Work out the finished part from the listing and answer in its coordinate system (mm). Round coordinates to 2 decimals unless told otherwise and drop trailing zeros. Order: outer loops, then holes, each group sorted by start corner. A loop starts at its lowest first (then second) coordinate and runs counter-clockwise, first axis right, second up. Notation, with made-up numbers: M -14.75,-38 L -4.75,-38 A24 cw -4.75,-17 Z; hole C -20.75,-18.75 d9. An arc over 180 degrees is marked long. Answer as a JSON object with one key per item and string values. Group by question number.
from build123d import *

# Parameters (mm, degrees)
SKETCH1_R           = 15
SKETCH1_R_2         = 13
SKETCH1_R_3         = 11.1
BOSS_EXTRUDE1_DEPTH = 6
SKETCH1_3_R         = 15
SKETCH1_3_R_2       = 13
CUT_EXTRUDE1_DEPTH  = 3.5
CHAMFER1_SIZE       = 2


with BuildPart() as part:
    # Sketch1 → Boss-Extrude1 (new, symmetric)
    # profile 1 of 2: a face of its own
    with BuildSketch(Plane.XY):
        Circle(SKETCH1_R)
        Circle(SKETCH1_R_2, mode=Mode.SUBTRACT)
    # profile 2 of 2: a face of its own
    with BuildSketch(Plane.XY):
        Circle(SKETCH1_R_2)
        Circle(SKETCH1_R_3, mode=Mode.SUBTRACT)
    extrude(amount=BOSS_EXTRUDE1_DEPTH, both=True)

    # Sketch1<3> → Cut-Extrude1 (cut, symmetric)
    with BuildSketch(Plane.XY):
        Circle(SKETCH1_3_R)
        Circle(SKETCH1_3_R_2, mode=Mode.SUBTRACT)
    extrude(amount=CUT_EXTRUDE1_DEPTH, both=True, mode=Mode.SUBTRACT)

    # Chamfer1
    chamfer1_edges = [part.edges().sort_by_distance(p)[0] for p in [
        (-15, 0, -3.5),
        (-15, 0, 3.5),
    ]]
    chamfer(chamfer1_edges, length=CHAMFER1_SIZE - 0.0001)  # a hair under: the kernel refuses the full size


solid = part.part
Item 1: Find section C-C (z = 1). Give the vertices of the cut face in (x, y), and give its area (3 significant figures).
Item 2: The mould has two halves that part along Z. Classify faces 1 (the cylindrical face through (-10.316, -7.91, -0.049)), 2 (the flat face through (2.2, 11.2, -6)), 3 (the cylindrical face through (-14.985, 0.66, -5.746)): +Z half, -Z half, draft (parallel to the pull), parting line (faces both ways), or undercut.
Item 3: Consider L1, parallel to Y at x = 0, z = -2.6; L2, parallel to Y at x = -4, z = -3; L3, parallel to Z at x = -12.5, y = -7.25. Determine where each line is inside the solid, lowest interval first.
Item 4: Each of these flat-tipped pins is pushed along its axis until it touches: pin 1 (1 mm diameter, centred on x = -10.5, z = -3.5, fed in from -Y); pin 2 (4 mm diameter, centred on y = 11.5, z = 4, fed in from +X); pin 3 (1.5 mm diameter, centred on x = 5.5, z = -2.5, fed in from +Y). Where does it stop, or does it pass through?
Item 5: Find section D-D (z = 4). Give the vertices of the cut face in (x, y).
Responses:
{
 "1": {"outline": "C 0,0 d26; hole C 0,0 d22.2", "area": "144 mm^2"},
 "2": {"face 1": "undercut", "face 2": "-Z half", "face 3": "draft"},
 "3": {"L1": "y = -13 to -11.1, 11.1 to 13", "L2": "y = -12.37 to -10.35, 10.35 to 12.37", "L3": "z = -6 to -4.95, 4.95 to 6"},
 "4": {"pin 1": "stops at y = -8.69", "pin 2": "stops at x = 11.02", "pin 3": "stops at y = 12.1"},
 "5": {"outline": "C 0,0 d27; hole C 0,0 d22.2"}
}
